CAD build for the part. Positions are in the model's coordinates, mm. Round coordinates to 2 decimals unless told otherwise and drop trailing zeros. Order: outer loops, then holes, each group sorted by start corner. A loop starts at its lowest first (then second) coordinate and runs counter-clockwise, first axis right, second up. Notation, with made-up numbers: M -28,9 L 23,9 A22 cw 23,15 Z; hole C 77.25,72 d7. An arc over 180 degrees is marked long. Answer as a JSON object with one key per item and string values.
Autodesk Fusion 360 part; units mm, degrees
sketch "Sketch1" plane through (0, 0, 0) normal (0, 0, 1) x (1, 0, 0)
  line L0 (4, 0) -> (96, 0)
  line L1 (100, 4) -> (100, 96)
  line L2 (96, 100) -> (4, 100)
  line L3 (0, 96) -> (0, 4)
  arc A0 (0, 4) -> (4, 0) centre (4, 4) ccw
  arc A1 (4, 100) -> (0, 96) centre (4, 96) ccw
  arc A2 (100, 96) -> (96, 100) centre (96, 96) ccw
  arc A3 (96, 0) -> (100, 4) centre (96, 4) ccw
  circle A4 centre (50, 49.9614) radius 44
  circle A5 centre (5, 95) radius 1.05
  circle A6 centre (95, 95) radius 1.05
  circle A7 centre (95, 5) radius 1.05
  circle A8 centre (5, 5) radius 1.05
  point P0 (100, 0)
  point P1 (0, 100)
  dimension "d1" = 100
  dimension "d2" = 100
  dimension "d3" = 4
  dimension "d4" = 4
  dimension "d5" = 4
  dimension "d6" = 4
  dimension "d7" = 88
  dimension "d8" = 2.1
  dimension "d9" = 2.1
  dimension "d10" = 2.1
  dimension "d11" = 2.1
extrude "Extrude1" add sketch "Sketch1" along normal blind 2
Item 1: Saw through at A-A on x = 50. List the corners of the cut face in (y, z).
Worked answers:
{"outline": "M 0,0 L 5.96,0 L 5.96,2 L 0,2 Z; M 93.96,0 L 100,0 L 100,2 L 93.96,2 Z"}
Item 2: Saw through at B-B on y = 15. List the corners of the cut face in (x, z), and give its area (3 significant figures).
Worked answers:
{"outline": "M 0,0 L 23.28,0 L 23.28,2 L 0,2 Z; M 76.72,0 L 100,0 L 100,2 L 76.72,2 Z", "area": "93.1 mm2"}
Item 3: Two-plate mould, pull along X, no slides. Class faces 1 (the flat face through (5, 51, 0)), 2 (the cylindrical face through (6.043, 48.027, 0.986)), 3 (the cylindrical face through (1.203, 1.141, 0.986)): released by +X, released by -X, zero draft, split by the parting line, or undercut.
Worked answers:
{"face 1": "zero draft", "face 2": "undercut", "face 3": "released by -X"}
Item 4: Saw through at C-C on z = 1.15. List the corners of the cut face in (x, y).
Worked answers:
{"outline": "M 0,4 A4 ccw 4,0 L 96,0 A4 ccw 100,4 L 100,96 A4 ccw 96,100 L 4,100 A4 ccw 0,96 Z; hole C 5,5 d2.1; hole C 5,95 d2.1; hole C 50,49.96 d88; hole C 95,5 d2.1; hole C 95,95 d2.1"}
Item 5: Wall check: line 1 along X through (y, z) = (95, 0.5); line 2 along X through (y, z) = (64, 1.25). Give the ranges that are in metal, low to high. Write a range as [from, to].
Worked answers:
{"line 1": "x = [0, 3.95], [6.05, 93.95], [96.05, 100]", "line 2": "x = [0, 8.3], [91.7, 100]"}
